Build history of the part. All positions in model axes, mm. A direction names the side the tool comes from. Round coordinates to 2 decimals unless told otherwise and drop trailing zeros. Loops run counter-clockwise (first coordinate to the right, second up) from the corner with the lowest first, then second, coordinate; pieces in that order, holes last. Notation, with made-up numbers: M 41,28.25 L 74,28.25 A22 ccw 74,64.25 Z; hole C 47,-39 d3. An arc over 180 degrees is marked long. One line per item, written item: value.
```python
from build123d import *

# Parameters (mm, degrees)
F1_R     = 6.15
F2_DEPTH = 61
F3_DEPTH = 61.001
F4_DEPTH = 2
F5_R     = 0.5


# Not quite as in the source:
# - two fillets or chamfers of one size are made in one step


with BuildPart() as f2:
    # F1 (on face) → F2 (new body)
    with BuildSketch(Plane.XZ):
        Circle(F1_R)
    extrude(amount=F2_DEPTH)


with BuildPart() as f2b:
    # F0 (on Front) → F2, piece 2 (new body)
    with BuildSketch(Plane.XZ):
        with BuildLine():
            ThreePointArc((11.8124997243, -2.1130192291), (11.9530330187, -1.0606609515), (12, 0))
            ThreePointArc((12, 0), (-1.0606609515, 11.9530330187), (-11.8124997243, -2.1130192291))
            Line((-11.8124997243, -2.1130192291), (-11.8124997243, 1))
            Line((-11.8124997243, 1), (11.8124997243, 1))
            Line((11.8124997243, 1), (11.8124997243, -2.1130192291))
        make_face()
        with BuildLine():
            Line((-11.8124997243, 1), (-11.8124997243, -2.1130192291))
            ThreePointArc((-11.8124997243, -2.1130192291), (0, -12), (11.8124997243, -2.1130192291))
            Line((11.8124997243, -2.1130192291), (11.8124997243, 1))
            Line((11.8124997243, 1), (-11.8124997243, 1))
        make_face()
        with BuildLine():
            ThreePointArc((11.8124997243, -2.1130192291), (0, -12), (-11.8124997243, -2.1130192291))
            Line((-11.8124997243, -2.1130192291), (-11.8124997243, -13))
            Line((-11.8124997243, -13), (11.8124997243, -13))
            Line((11.8124997243, -13), (11.8124997243, -2.1130192291))
        make_face()
    extrude(amount=F2_DEPTH)


with BuildPart() as f3_tool:
    # F3 (cut, through all): a face of the model
    f3_faces = [f2.part.faces().sort_by_distance(p)[0] for p in [
        (0, -61, 0),
    ]]
    extrude(f3_faces, amount=-F3_DEPTH)


with BuildPart() as f2_1:
    add(f2.part)

    # F3: cut by f3_tool
    add(f3_tool.part, mode=Mode.SUBTRACT)


with BuildPart() as f2b_1:
    add(f2b.part)

    # F3: cut by f3_tool
    add(f3_tool.part, mode=Mode.SUBTRACT)

    # F4 (add): a face of the model
    f4_faces = [f2b_1.faces().sort_by_distance(p)[0] for p in [
        (0, -30.5, -13),
    ]]
    extrude(f4_faces, amount=F4_DEPTH)

    # F5
    f5_edges = [f2b_1.edges().sort_by_distance(p)[0] for p in [
        (0, -61, 12),
        (-11.8125, -61, -8.55651),
        (11.8125, -61, -8.55651),
        (11.8125, 0, -8.55651),
        (-11.8125, 0, -8.55651),
        (0, 0, 12),
        (-11.8125, -30.5, -15),
        (0, 0, -15),
        (11.8125, -30.5, -15),
        (0, -61, -15),
    ]]
    fillet(f5_edges, radius=F5_R)


solid = f2b_1.part
```
Item 1: Slice it at B-B, the plane z = -3. Give the cut face in (x, y), and give its area (3 significant figures).
Check values:
outline: M -11.81,-60.5 A0.5 ccw -11.31,-61 L -5.37,-61 L -5.37,0 L -11.31,0 A0.5 ccw -11.81,-0.5 Z; M 5.37,-61 L 11.31,-61 A0.5 ccw 11.81,-60.5 L 11.81,-0.5 A0.5 ccw 11.31,0 L 5.37,0 Z
area: 786 mm2
Item 2: Wall check: line 1 along Z through (x, y) = (0, -34.5); line 2 along X through (y, z) = (-24.5, -13.5); line 3 along X through (y, z) = (-38.5, -4). Give the ranges that are in metal, low to high.
Check values:
line 1: z = -15 to -6.15, 6.15 to 12
line 2: x = -11.81 to 11.81
line 3: x = -11.81 to -4.67, 4.67 to 11.81
Item 3: Drop flat-ended pins along their axis: P1, Ø8, axis at y = -15.5, z = 4.5, coming from the -X side; P2, Ø3, axis at y = -40.5, z = 4.5, coming from the +X side; P3, Ø13.5, axis at y = -35.5, z = -9, coming from the +X side. Give the stop position or say it passes through.
Check values:
P1: stops at x = -11.99
P2: stops at x = 11.62
P3: stops at x = 11.81
Item 4: Which spindle directions (+Z, -Z, +X, -X, +Y, -Y) get a long thin tool onto all of the face, cutting with end or side? Do faces 4 (the face through (-11.812, -30, -8)), 5 (the face through (11.812, -30, -8)), 6 (the face through (0, -61, -7)). Say none if no direction does.
Check values:
face 4: -Z, -X, +Y, -Y
face 5: -Z, +X, +Y, -Y
face 6: +Z, -Z, +X, -X, -Y
Item 5: Slice it at C-C, the plane z = -9. Give the cut face in (x, y).
Check values:
outline: M -11.81,-60.5 A0.5 ccw -11.31,-61 L 11.31,-61 A0.5 ccw 11.81,-60.5 L 11.81,-0.5 A0.5 ccw 11.31,0 L -11.31,0 A0.5 ccw -11.81,-0.5 Z
Item 6: Slice it at A-A, the plane y = -22. Give the cut face in (x, z), and give its area (3 significant figures).
Check values:
outline: M -11.81,-14.5 A0.5 ccw -11.31,-15 L 11.31,-15 A0.5 ccw 11.81,-14.5 L 11.81,-2.11 A12 ccw long -11.81,-2.11 Z; hole C 0,0 d12.3
area: 462 mm2
Item 7: Pull direction Z, two halves, no side cores. Call faces 1 (the face through (0, -30, -15)), 2 (the face through (-1.333, -30.927, -6.004)), 3 (the face through (0, 0, -7)): pulls with the +Z half, pulls with the -Z half, needs draft (parallel to the pull), parting line crosses it, or undercut.
Check values:
face 1: pulls with the -Z half
face 2: undercut
face 3: needs draft
